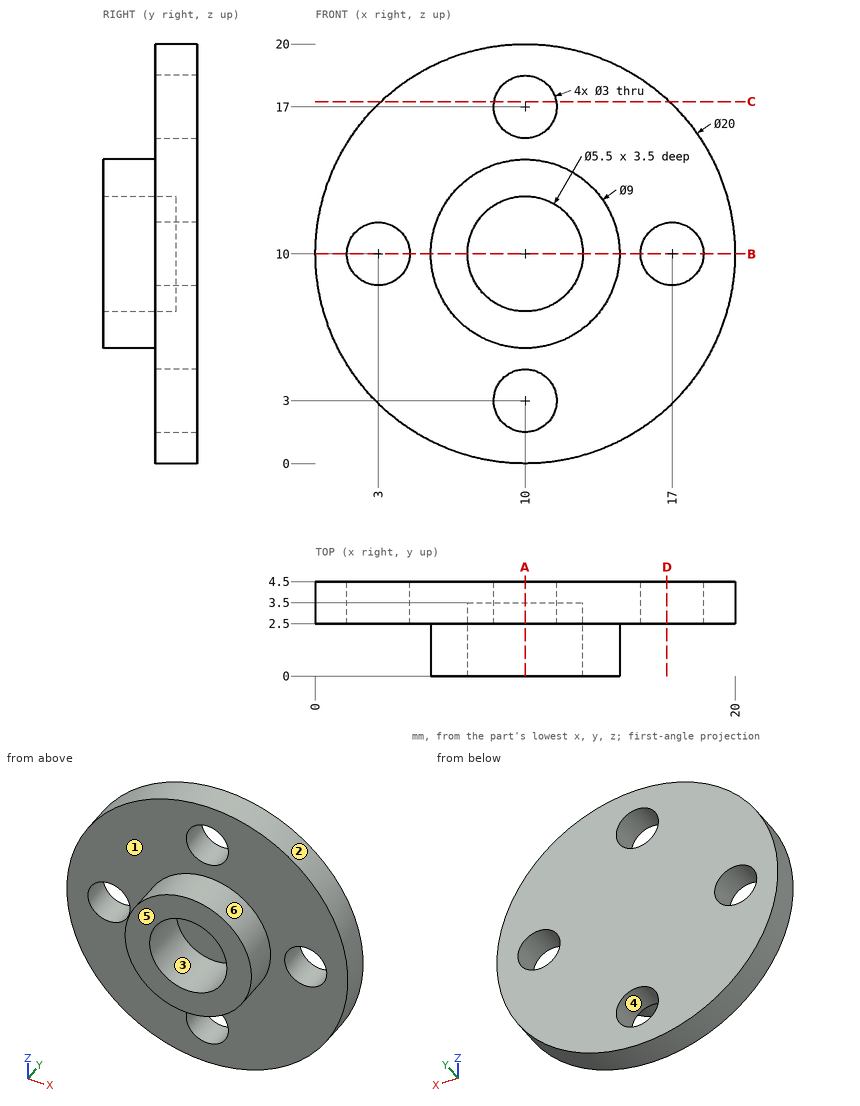
Input: dimensioned drawing with shaded views. Units: mm. Origin: part minimum x, y, z. A direction names the side the tool comes from. Give positions to 0.01 mm unless a question says otherwise; leave off trailing zeros. Loops run counter-clockwise (first coordinate to the right, second up) from the corner with the lowest first, then second, coordinate; pieces in that order, holes last. Notation, with made-up numbers: (66.25, 76.5) -> (111.25, 76.5) arc R25 cw to (111.25, 114.5) -> close; hole circle Ø11 at (68.25, 0). An arc over 180 degrees is marked (long way). Return JSON: item names as keys, results as strings.
Item 1: Section A-A, the plane x = 10. Output: boundary loops of the cut face in (y, z).
Filled in:
{"outline": "(0, 5.5) -> (2.5, 5.5) -> (2.5, 4.5) -> (4.5, 4.5) -> (4.5, 15.5) -> (2.5, 15.5) -> (2.5, 14.5) -> (0, 14.5) -> (0, 12.75) -> (3.5, 12.75) -> (3.5, 7.25) -> (0, 7.25) -> close; (2.5, 0) -> (4.5, 0) -> (4.5, 1.5) -> (2.5, 1.5) -> close; (2.5, 18.5) -> (4.5, 18.5) -> (4.5, 20) -> (2.5, 20) -> close"}
Item 2: Section D-D, the plane x = 16.75. Output: boundary loops of the cut face in (y, z).
Filled in:
{"outline": "(2.5, 2.62) -> (4.5, 2.62) -> (4.5, 8.52) -> (2.5, 8.52) -> close; (2.5, 11.48) -> (4.5, 11.48) -> (4.5, 17.38) -> (2.5, 17.38) -> close"}
Item 3: Pin query (flat end, axial travel): P1, Ø4, axis at x = 10, z = 3, coming from the -Y side. Return the tip coordinate at first contact, or that it passes through.
Filled in:
{"P1": "y = 2.5"}
Item 4: Section C-C, the plane z = 17.25. Output: boundary loops of the cut face in (x, y).
Filled in:
{"outline": "(3.11, 2.5) -> (8.52, 2.5) -> (8.52, 4.5) -> (3.11, 4.5) -> close; (11.48, 2.5) -> (16.89, 2.5) -> (16.89, 4.5) -> (11.48, 4.5) -> close"}
Item 5: Line query: line 1 (X direction, y = 3.25, z = 10.5); line 2 (X direction, y = 0.7, z = 10); line 3 (Y direction, x = 10.5, z = 18.5). Output: solid intervals per line, ascending.
Filled in:
{"line 1": "0.01 to 1.59, 4.41 to 7.3, 12.7 to 15.59, 18.41 to 19.99", "line 2": "5.5 to 7.25, 12.75 to 14.5", "line 3": "2.5 to 4.5"}
Item 6: Access query for the marked faces 1 and 2. Directions: +Z, -Z, +X, -X, +Y, -Y. A direction counts if a zero-diameter tool reaches every point of the face in a straight line with its end or side. Return the directions, or none.
Filled in:
{"face 1": "-Y", "face 2": "+Y, -Y"}
Item 7: Mould query, pull axis X, two halves, no side actions, for the marked faces 3, 4, 5 and 6. Classes: released by +X, released by -X, zero draft, split by the parting line, or undercut.
Filled in:
{"face 3": "undercut", "face 4": "undercut", "face 5": "zero draft", "face 6": "split by the parting line"}
Item 8: Section B-B, the plane z = 10. Output: boundary loops of the cut face in (x, y), plus the area to 4 significant figures.
Filled in:
{"outline": "(0, 2.5) -> (1.5, 2.5) -> (1.5, 4.5) -> (0, 4.5) -> close; (4.5, 2.5) -> (5.5, 2.5) -> (5.5, 0) -> (7.25, 0) -> (7.25, 3.5) -> (12.75, 3.5) -> (12.75, 0) -> (14.5, 0) -> (14.5, 2.5) -> (15.5, 2.5) -> (15.5, 4.5) -> (4.5, 4.5) -> close; (18.5, 2.5) -> (20, 2.5) -> (20, 4.5) -> (18.5, 4.5) -> close", "area": "31.25 mm^2"}
